```python
from build123d import *

# Parameters (mm, degrees)
F0_W     = 50.8
F0_H     = 50.8
F1_DEPTH = 133.35
F2_W     = 44.45
F2_H     = 44.45
F3_DEPTH = 876.3
F4_R     = 9.525
F6_D     = 12.7
F6_DEPTH = 127


with BuildPart() as f1:
    # F0 (on Right) → F1 (new body)
    with BuildSketch(Plane.YZ):
        with Locations((25.4, 25.4)):
            Rectangle(F0_W, F0_H)
    extrude(amount=-F1_DEPTH)

    # F2 (on face) → F3 (cut)
    with BuildSketch(Plane.YZ):
        with Locations((25.4, 25.4)):
            Rectangle(F2_W, F2_H)
    extrude(amount=-F3_DEPTH, mode=Mode.SUBTRACT)

    # F4
    f4_edges = [f1.edges().sort_by_distance(p)[0] for p in [
        (-66.675, 3.175, 3.175),
        (-66.675, 47.625, 3.175),
        (-66.675, 47.625, 47.625),
        (-66.675, 3.175, 47.625),
        (-66.675, 50.8, 0),
        (-66.675, 50.8, 50.8),
        (-66.675, 0, 50.8),
        (-66.675, 0, 0),
    ]]
    fillet(f4_edges, radius=F4_R)

    # F6
    with Locations(Plane(origin=(0, 50.8, 0), x_dir=(-1, 0, 0), z_dir=(0, 1, 0))):
        with Locations((120.65, 31.75), (95.25, 31.75), (38.1, 31.75), (12.7, 31.75)):
            Hole(F6_D / 2, depth=F6_DEPTH)


solid = f1.part
```
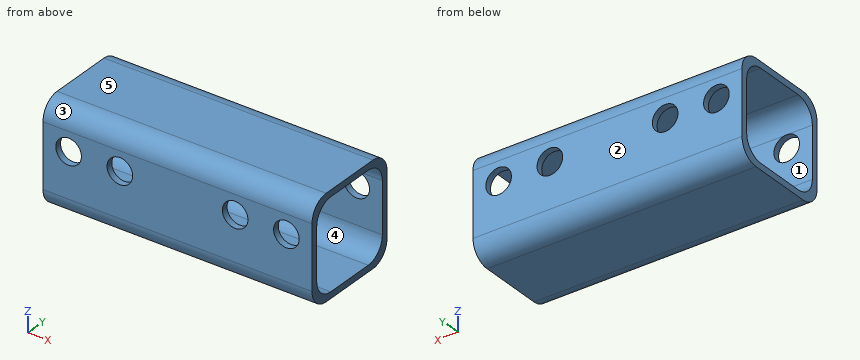
Could you check a few things on this model? Use its own coordinates, in mm. Face numbers are marked on the shaded views. A direction names the side the tool comes from. Coordinates: 2 decimals unless noted, no trailing zeros. Loops run counter-clockwise (first coordinate to the right, second up) from the corner with the lowest first, then second, coordinate; pieces in that order, holes last.
1) Which directions (+Z, -Z, +X, -X, +Y, -Y) give clear straight access to the entire face, cutting with the end or side of a thin tool? Please do the marked faces 4 and 5.
Reported:
face 4: +X, -X
face 5: +Z, +X, -X, +Y, -Y
2) Imagine slicing it at D-D (z = 31.75). State how many separate pieces and enclosed holes the cut face has, and give its area (3 significant figures).
Reported:
separate pieces: 10
enclosed holes: 0
area: 524 mm2
3) Thinking about a two-plate mould opening in Z: for the marked faces 1, 2 and 3, which applies, released by +Z, released by -Z, zero draft, split by the parting line, or undercut?
Reported:
face 1: undercut
face 2: zero draft
face 3: released by +Z
4) Imagine slicing it at A-A (y = 25). List the corners of the cut face in (x, z) for me (3 decimals), and give its area (3 significant figures).
Reported:
outline: (-133.35, 0) - (0, 0) - (0, 3.175) - (-133.35, 3.175) - close; (-133.35, 47.625) - (0, 47.625) - (0, 50.8) - (-133.35, 50.8) - close
area: 847 mm2
5) Please list where these lines run through material, in increasing order: line 1 along X through (y, z) = (49.35, 31.75); line 2 along Z through (x, y) = (-17, 35) (3 decimals).
Reported:
line 1: x = -133.35 to -127, -114.3 to -101.6, -88.9 to -44.45, -31.75 to -19.05, -6.35 to 0
line 2: z = 0 to 3.175, 47.625 to 50.8
6) Imagine slicing it at C-C (x = -56). List the corners of the cut face in (y, z) for me (3 decimals), and give its area (3 significant figures).
Reported:
outline: (0, 9.525) arc R9.525 ccw to (9.525, 0) - (41.275, 0) arc R9.525 ccw to (50.8, 9.525) - (50.8, 41.275) arc R9.525 ccw to (41.275, 50.8) - (9.525, 50.8) arc R9.525 ccw to (0, 41.275) - close; hole (3.175, 12.7) arc R9.525 ccw to (12.7, 3.175) - (38.1, 3.175) arc R9.525 ccw to (47.625, 12.7) - (47.625, 38.1) arc R9.525 ccw to (38.1, 47.625) - (12.7, 47.625) arc R9.525 ccw to (3.175, 38.1) - close
area: 605 mm2
7) Will these pins go through, and if not, where does the flat tip stop? pin 1 Ø10 at (x, z) = (-12.7, 31.75) entering from -Y; pin 2 Ø10 at (y, z) = (45, 36) entering from +X.
Reported:
pin 1: passes through
pin 2: stops at x = 0
